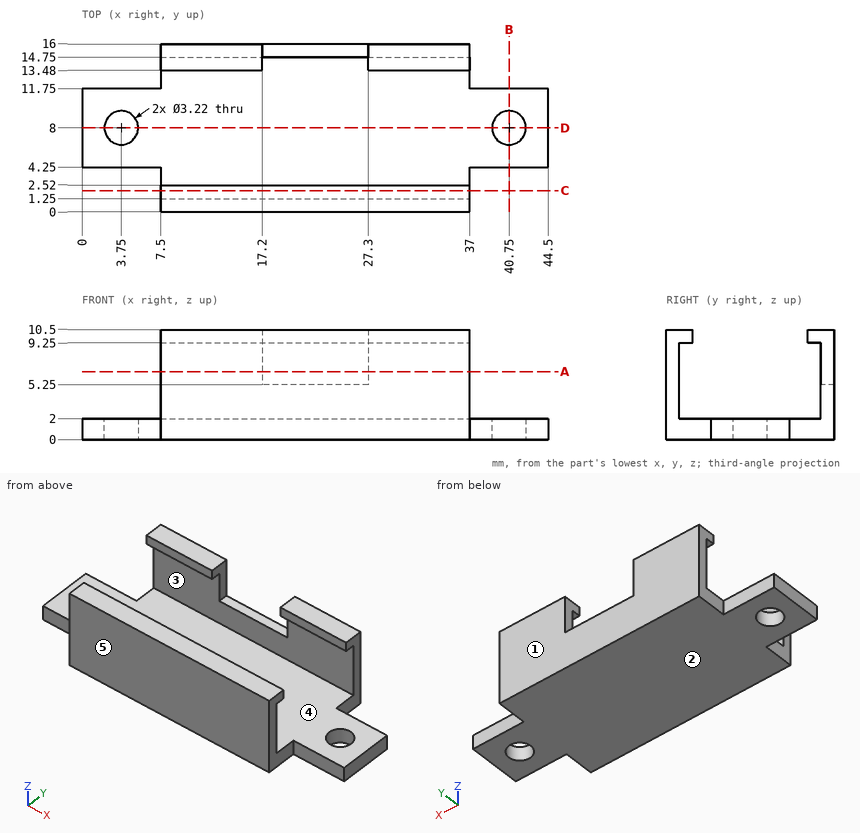
Could you check a few things on this drawing? It's one solid part, dimensions in mm from its lowest x, y, z. A direction names the side the tool comes from. Round coordinates to 2 decimals unless told otherwise and drop trailing zeros. Loops run counter-clockwise (first coordinate to the right, second up) from the corner with the lowest first, then second, coordinate; pieces in that order, holes last. Notation, with made-up numbers: (68.5, 35) -> (73.5, 35) arc R28 ccw to (73.5, 54) -> close; hole circle Ø7 at (88.25, 74.25). An arc over 180 degrees is marked (long way). Answer as CSV lines item,"result".
1. Thinking about a two-plate mould opening in Z: for the marked faces 1, 2 and 3, which applies, released by +Z, released by -Z, zero draft, split by the parting line, or undercut?
Final values:
face 1,"zero draft"
face 2,"released by -Z"
face 3,"undercut"
2. If we section it at D-D on y = 8: Please give me the cut outline in (x, z), plus the area to 3 significant figures.
Final values:
outline,"(0, 0) -> (2.14, 0) -> (2.14, 2) -> (0, 2) -> close; (5.36, 0) -> (39.14, 0) -> (39.14, 2) -> (5.36, 2) -> close; (42.36, 0) -> (44.5, 0) -> (44.5, 2) -> (42.36, 2) -> close"
area,"76.1 mm^2"
3. If we section it at B-B on x = 40.75: Please give me the cut outline in (y, z).
Final values:
outline,"(4.25, 0) -> (6.39, 0) -> (6.39, 2) -> (4.25, 2) -> close; (9.61, 0) -> (11.75, 0) -> (11.75, 2) -> (9.61, 2) -> close"
4. If I drill on L1, parallel to Z at x = 9, y = 2; L2, parallel to Y at x = 3.75, z = 1.4; L3, parallel to Y at x = 36.5, z = 4.5, over which ranges is the centre line in solid material (lowest first)?
Final values:
L1,"z = 0 to 2, 9.25 to 10.5"
L2,"y = 4.25 to 6.39, 9.61 to 11.75"
L3,"y = 0 to 1.25, 14.75 to 16"
5. If we section it at A-A on z = 6.5: Please give me the cut outline in (x, y), plus the area to 3 significant figures.
Final values:
outline,"(7.5, 0) -> (37, 0) -> (37, 1.25) -> (7.5, 1.25) -> close; (7.5, 14.75) -> (17.2, 14.75) -> (17.2, 16) -> (7.5, 16) -> close; (27.3, 14.75) -> (37, 14.75) -> (37, 16) -> (27.3, 16) -> close"
area,"61.1 mm^2"
6. For pin 1 (3.5 mm diameter, centred on y = 1.5, z = 5, fed in from -X); pin 2 (5 mm diameter, centred on y = 3.5, z = 5, fed in from +X); pin 3 (1.6 mm diameter, centred on x = 3, z = 1, fed in from +Y), each with a flat end and sliding along its axis, tell me the tip position at first contact or that it passes through.
Final values:
pin 1,"stops at x = 7.5"
pin 2,"stops at x = 37"
pin 3,"stops at y = 11.75"
7. If we section it at C-C on y = 2: Please give me the cut outline in (x, z).
Final values:
outline,"(7.5, 0) -> (37, 0) -> (37, 2) -> (7.5, 2) -> close; (7.5, 9.25) -> (37, 9.25) -> (37, 10.5) -> (7.5, 10.5) -> close"
8. Which directions (+Z, -Z, +X, -X, +Y, -Y) give clear straight access to the entire face, cutting with the end or side of a thin tool? Please do the marked faces 4 and 5.
Final values:
face 4,"+X, -X"
face 5,"+Z, -Z, +X, -X, -Y"
